Geometry: final body of the model. Coordinates: model frame, mm. A direction names the side the tool comes from. Give positions to 0.01 mm unless a question says otherwise; leave off trailing zeros. Loops run counter-clockwise (first coordinate to the right, second up) from the corner with the lowest first, then second, coordinate; pieces in that order, holes last. Notation, with made-up numbers: M 56.25,52 L 101.25,52 A21 cw 101.25,79 Z; hole C 5.25,10.5 d6. An arc over 180 degrees is marked long. One line per question, with ' | ' between items. Start each with the question number.
Autodesk Inventor part; units mm, degrees
ref_plane "Work Plane2" through (-40.9959, 0.8639, 22.2359) normal (0, 0, 1) x (1, 0, 0)
ref_plane "YZ Plane" through (0, 0, 0) normal (1, 0, 0) x (0, 1, 0)
ref_plane "XZ Plane" through (0, 0, 0) normal (0, 1, 0) x (-1, 0, 0)
ref_plane "Work Plane1" through (0, 0, 10) normal (0, 0, 1) x (1, 0, 0)
sketch "Sketch1" plane through (0, 0, 10) normal (0, 0, 1) x (1, 0, 0)
  line L0 (-4.0299, -0.3538) -> (-2.2322, 1.4439) construction
  arc A0 (-1.4439, 2.2322) -> (-2.2322, 1.4439) centre (-0.9299, 0.9299) ccw construction
  line L1 (-1.4439, 2.2322) -> (0.3538, 4.0299) construction
  line L2 (-37.8299, 42.8299) -> (-37.8299, 37.8299) construction
  line L3 (-37.8299, 37.8299) -> (-42.9208, 37.8299) construction
  line L4 (-37.8299, 42.2137) -> (-37.8299, 45.8299) construction
  line L5 (-37.8299, 45.8299) -> (-4.0299, 45.8299) construction
  line L6 (-4.0299, 45.8299) -> (-4.0299, 42.2137) construction
  line L7 (-4.0299, 4.0299) -> (0.3538, 4.0299)
  circle A1 centre (-20.9299, 20.9299) radius 17.5
  line L8 (-20.9299, 58.9723) -> (17.1124, 20.9299) construction
  line L9 (17.1124, 20.9299) -> (-20.9299, -17.1124) construction
  line L10 (-20.9299, -17.1124) -> (-58.9723, 20.9299) construction
  line L11 (-58.9723, 20.9299) -> (-20.9299, 58.9723) construction
  line L12 (-20.9299, 58.9723) -> (-20.9299, -17.1124) construction
  line L13 (17.1124, 20.9299) -> (-58.9723, 20.9299) construction
  line L14 (-20.9299, 58.9723) -> (32.8701, 58.9723) construction
  line L15 (-43.4299, 43.4299) -> (1.5701, 43.4299) construction
  line L16 (1.5701, 43.4299) -> (1.5701, -1.5701) construction
  line L17 (1.5701, -1.5701) -> (-43.4299, -1.5701) construction
  line L18 (-43.4299, -1.5701) -> (-43.4299, 43.4299) construction
  line L19 (-43.4299, 43.4299) -> (1.5701, -1.5701) construction
  line L20 (1.5701, 43.4299) -> (-43.4299, -1.5701) construction
  line L21 (-43.4299, 5.3876) -> (-43.4299, 36.4723)
  line L22 (-43.4299, 36.4723) -> (-36.4723, 43.4299)
  line L23 (-36.4723, 43.4299) -> (-5.3876, 43.4299)
  line L24 (-5.3876, 43.4299) -> (1.5701, 36.4723)
  line L25 (1.5701, 36.4723) -> (1.5701, 5.3876)
  line L26 (1.5701, 5.3876) -> (-5.3876, -1.5701)
  line L27 (-5.3876, -1.5701) -> (-36.4723, -1.5701)
  line L28 (-36.4723, -1.5701) -> (-43.4299, 5.3876)
  line L29 (-4.0299, 42.2137) -> (-37.8299, 42.2137)
  line L30 (-4.0299, -0.3538) -> (-4.0299, 4.0299)
  point P0 (-37.8299, 4.0299)
  point P1 (-20.9299, 20.9299)
  dimension "d18" = 53.8
  dimension "d19" = 45
  dimension "d20" = 53.8
  dimension "d21" = 45
  dimension "d22" = 45
extrude "Extrusion1" add sketch "Sketch1" along normal blind 8
sketch "Sketch2" plane through (0, 0, 18) normal (0, 0, 1) x (1, 0, 0)
  circle A0 centre (-35.9299, 35.9299) radius 3.0099 construction
  circle A1 centre (-5.93, 35.9299) radius 3.0099 construction
  circle A2 centre (-5.93, 5.93) radius 3.0099 construction
  circle A3 centre (-35.9299, 5.93) radius 3.0099 construction
  circle A4 centre (-35.9299, 35.9299) radius 3.05
  circle A5 centre (-5.93, 35.9299) radius 3.05
  circle A6 centre (-5.93, 5.93) radius 3.05
  circle A7 centre (-35.9299, 5.93) radius 3.05
  point P0 (0, 0)
  dimension "d30" = 6.1
  dimension "d31" = 6.1
  dimension "d32" = 6.1
  dimension "d33" = 6.1
ref_plane "Work Plane2" through (-40.9959, 0.8639, 22.2359) normal (0, 0, 1) x (1, 0, 0)
extrude "Extrusion2" cut sketch "Sketch2" against normal through all
sketch "Sketch3" plane through (0, 0, 10) normal (0, 0, -1) x (-1, 0, 0)
  line L0 (37.8299, -0.4701) -> (37.8299, 4.0299) construction
  line L1 (4.0299, 4.0299) -> (4.0299, -0.4701) construction
  line L2 (37.8299, -0.4701) -> (37.8299, 1.1886) construction
  line L3 (4.0299, -3.9701) -> (4.0299, -0.3538) construction
  line L4 (45.8299, 4.0299) -> (42.2137, 4.0299) construction
  line L5 (-0.3538, 4.0299) -> (-3.9701, 4.0299) construction
  line L6 (-3.9701, 37.8299) -> (-0.3538, 37.8299) construction
  line L7 (4.0299, 42.2137) -> (4.0299, 45.8299) construction
  line L8 (37.8299, 45.8299) -> (37.8299, 42.2137) construction
  line L9 (42.2137, 37.8299) -> (45.8299, 37.8299) construction
  line L10 (40.4657, 37.7299) -> (45.8299, 37.7299)
  line L11 (45.8299, 37.7299) -> (45.8299, 4.1299)
  line L12 (45.8299, 4.1299) -> (40.4657, 4.1299)
  line L13 (40.4657, 4.1299) -> (40.4657, 37.7299)
  line L14 (37.7299, 2.4952) -> (4.1299, 2.4952)
  line L15 (4.1299, 2.4952) -> (4.1299, -3.9701)
  line L16 (4.1299, -3.9701) -> (37.7299, -3.9701)
  line L17 (37.7299, -3.9701) -> (37.7299, 2.4952)
  line L18 (1.8946, 4.1299) -> (-3.9701, 4.1299)
  line L19 (-3.9701, 4.1299) -> (-3.9701, 37.7299)
  line L20 (-3.9701, 37.7299) -> (1.8946, 37.7299)
  line L21 (1.8946, 37.7299) -> (1.8946, 4.1299)
  line L22 (4.1299, 40.7326) -> (37.7299, 40.7326)
  line L23 (37.7299, 40.7326) -> (37.7299, 45.8299)
  line L24 (37.7299, 45.8299) -> (4.1299, 45.8299)
  line L25 (4.1299, 45.8299) -> (4.1299, 40.7326)
  point P0 (0, 0)
  dimension "d23" = 0.1
  dimension "d24" = 0.1
  dimension "d25" = 0.1
  dimension "d26" = 0.1
  dimension "d27" = 0.1
extrude "Extrusion3" add sketch "Sketch3" against normal up to surface (8 mm away)
sketch "Sketch4" plane through (0, 0, 18) normal (0, 0, 1) x (1, 0, 0)
  line L0 (3.9701, 4.1299) -> (0.3124, 4.1299)
  line L1 (3.9701, 37.7299) -> (3.9701, 4.1299)
  line L2 (0.3124, 37.7299) -> (3.9701, 37.7299)
  line L3 (0.3124, 37.7299) -> (-4.1299, 42.1723)
  line L4 (-4.1299, 45.8299) -> (-4.1299, 42.1723)
  line L5 (-37.7299, 45.8299) -> (-4.1299, 45.8299)
  line L6 (-37.7299, 42.1723) -> (-37.7299, 45.8299)
  line L7 (-37.7299, 42.1723) -> (-42.1723, 37.7299)
  line L8 (-45.8299, 37.7299) -> (-42.1723, 37.7299)
  line L9 (-45.8299, 4.1299) -> (-45.8299, 37.7299)
  line L10 (-42.1723, 4.1299) -> (-45.8299, 4.1299)
  line L11 (-42.1723, 4.1299) -> (-37.7299, -0.3124)
  line L12 (-37.7299, -3.9701) -> (-37.7299, -0.3124)
  line L13 (-4.1299, -3.9701) -> (-37.7299, -3.9701)
  line L14 (-4.1299, -0.3124) -> (-4.1299, -3.9701)
  line L15 (-4.1299, -0.3124) -> (0.3124, 4.1299)
  circle A0 centre (-20.9299, 20.9299) radius 17.5
  circle A1 centre (-35.9299, 5.93) radius 3.05
  circle A2 centre (-5.93, 35.9299) radius 3.05
  circle A3 centre (-35.9299, 35.9299) radius 3.05
  circle A4 centre (-5.93, 5.93) radius 3.05
  line L16 (-3.9799, 45.9799) -> (-3.9799, 42.2344)
  line L17 (-3.9799, 42.2344) -> (0.3745, 37.8799)
  line L18 (0.3745, 37.8799) -> (4.1201, 37.8799)
  line L19 (4.1201, 37.8799) -> (4.1201, 3.9799)
  line L20 (4.1201, 3.9799) -> (0.3745, 3.9799)
  line L21 (0.3745, 3.9799) -> (-3.9799, -0.3745)
  line L22 (-3.9799, -0.3745) -> (-3.9799, -4.1201)
  line L23 (-3.9799, -4.1201) -> (-37.8799, -4.1201)
  line L24 (-37.8799, -4.1201) -> (-37.8799, -0.3745)
  line L25 (-37.8799, -0.3745) -> (-42.2344, 3.9799)
  line L26 (-42.2344, 3.9799) -> (-45.9799, 3.9799)
  line L27 (-45.9799, 3.9799) -> (-45.9799, 37.8799)
  line L28 (-45.9799, 37.8799) -> (-42.2344, 37.8799)
  line L29 (-42.2344, 37.8799) -> (-37.8799, 42.2344)
  line L30 (-37.8799, 42.2344) -> (-37.8799, 45.9799)
  line L31 (-37.8799, 45.9799) -> (-3.9799, 45.9799)
  point P0 (0, 0)
  dimension "d34" = 0.15
extrude "Extrusion4" add sketch "Sketch4" against normal up to surface (8 mm away) contours L16 L17 L18 L19 L20 L21 L22 L23 L24 L25 L26 L27 L28 L29 L30 L31
properties part number "50_Cube_Insert_Thorlabs"
Q1. Section C-C, the plane x = -6.5. Output: boundary loops of the cut face in (y, z).
Q2. Section A-A, the plane x = -25. Output: boundary loops of the cut face in (y, z), plus the area to 3 significant figures.
Q3. Section D-D, the plane y = 5.93. Output: boundary loops of the cut face in (x, z).
Q4. Draft query along X for faces 1 (the cylindrical face through (-4.24, 15.67, 13.94)), 2 (the flat face through (-3.98, 44, 14)), 3 (the flat face through (-16, 38, 10)). Return one class per face: released by +X, released by -X, zero draft, split by the parting line, or undercut.
Q5. Set-up query: faces 4 (the flat face through (-44, 37.88, 14)), 5 (the flat face through (2, 3.98, 14)), 6 (the flat face through (-21, 45.98, 14)), 7 (the flat face through (-44, 3.98, 14)), 8 (the flat face through (2, 37.88, 14)). Return all of +Z, -Z, +X, -X, +Y, -Y with unobstructed straight access to the full face (end or side cutting, diameter ignored); none if empty.
Q6. Section B-B, the plane y = 14. Output: boundary loops of the cut face in (x, z), plus the area to 3 significant figures.
Q7. Contact query for flat-ended pins moving along their axis: pin 1 (1.9 mm diameter, centred on x = 2, z = 15.5, fed in from -Y); pin 2 (4 mm diameter, centred on y = 44, z = 15, fed in from +X); pin 3 (1.1 mm diameter, centred on y = -2.5, z = 14, fed in from -X). Output: stop coordinate, or through.
Q8. Material intervals for L1, parallel to Y at x = -5.93, z = 12; L2, parallel to X at y = 21, z = 16.5; L3, parallel to Y at x = -6.5, z = 13.5, sorted ascending.
Model answer:
1) outline: M -4.12,10 L 2.93,10 L 2.93,18 L -4.12,18 Z; M 8.93,10 L 11.03,10 L 11.03,18 L 8.93,18 Z; M 30.83,10 L 32.93,10 L 32.93,18 L 30.83,18 Z; M 38.93,10 L 45.98,10 L 45.98,18 L 38.93,18 Z
2) outline: M -4.12,10 L 3.91,10 L 3.91,18 L -4.12,18 Z; M 37.95,10 L 45.98,10 L 45.98,18 L 37.95,18 Z | area: 128 mm^2
3) outline: M -45.98,10 L -38.98,10 L -38.98,18 L -45.98,18 Z; M -32.88,10 L -29.94,10 L -29.94,18 L -32.88,18 Z; M -11.92,10 L -8.98,10 L -8.98,18 L -11.92,18 Z; M -2.88,10 L 4.12,10 L 4.12,18 L -2.88,18 Z
4) face 1: undercut | face 2: released by +X | face 3: zero draft
5) face 4: +Z, -Z, -X, +Y | face 5: +Z, -Z, +X, -Y | face 6: +Z, -Z, +X, -X, +Y | face 7: +Z, -Z, -X, -Y | face 8: +Z, -Z, +X, +Y
6) outline: M -45.98,10 L -37,10 L -37,18 L -45.98,18 Z; M -4.86,10 L 4.12,10 L 4.12,18 L -4.86,18 Z | area: 144 mm^2
7) pin 1: stops at y = 3.98 | pin 2: stops at x = -3.75 | pin 3: stops at x = -37.88
8) L1: y = -4.12 to 2.88, 8.98 to 11.92, 29.94 to 32.88, 38.98 to 45.98 | L2: x = -45.98 to -38.43, -3.43 to 4.12 | L3: y = -4.12 to 2.93, 8.93 to 11.03, 30.83 to 32.93, 38.93 to 45.98
